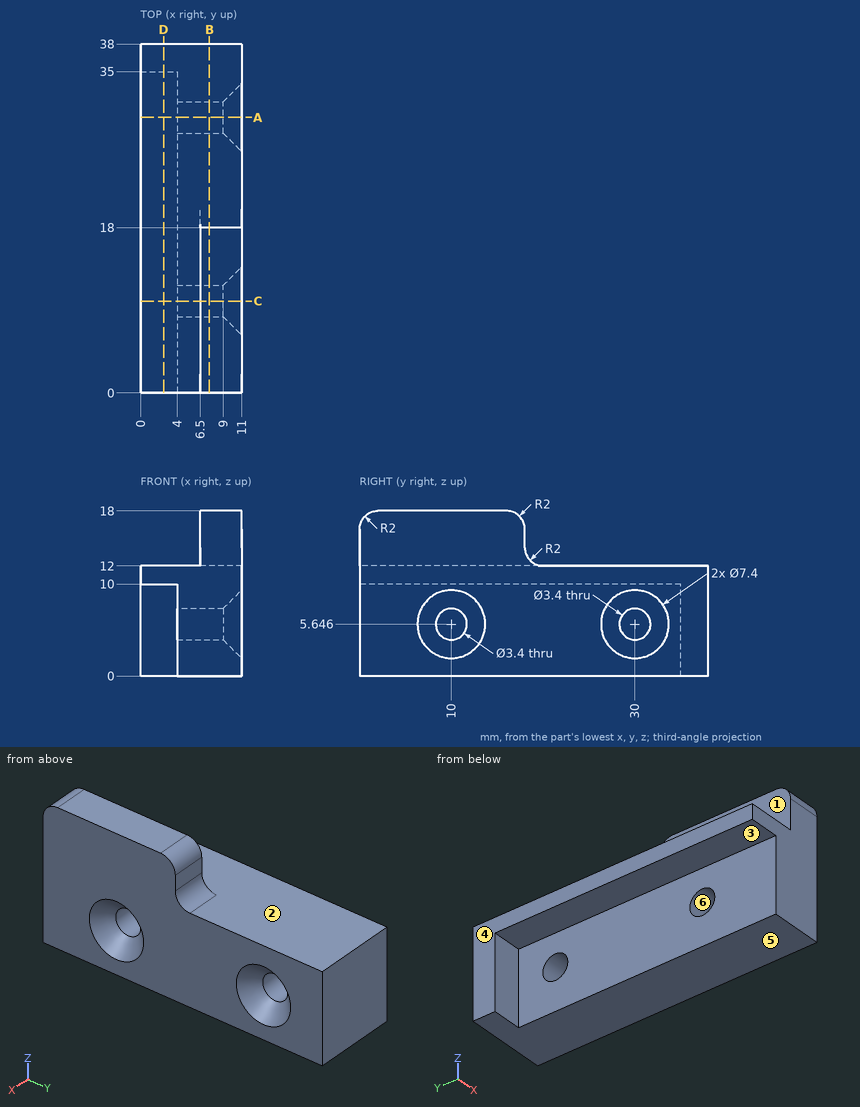
Geometry: see drawing. Coordinates: mm, zero at the bounding-box minimum. A direction names the side the tool comes from. Coordinates: 2 decimals unless noted, no trailing zeros. Loops run counter-clockwise (first coordinate to the right, second up) from the corner with the lowest first, then second, coordinate; pieces in that order, holes last. Notation, with made-up numbers: M 35.25,55 L 82.25,55 A22 ccw 82.25,67 Z; hole C 51,-34 d3. An arc over 180 degrees is marked long. Answer in a Markdown table with one row per item.
Q1. Set-up query: the marked faces 1, 2 and 3. Return all of +Z, -Z, +X, -X, +Y, -Y with unobstructed straight access to the full face (end or side cutting, diameter ignored); none if empty.
Answers below:
| item | result |
|---|---|
| face 1 | +Z, -X, +Y, -Y |
| face 2 | +Z, -X, +Y |
| face 3 | -Z, -X, -Y |
Q2. Section B-B on x = 7.5. Return the cut outline in (y, z) (1 decimal).
Answers below:
| item | result |
|---|---|
| outline | M 0,0 L 38,0 L 38,12 L 20,12 A2 cw 18,14 L 18,16 A2 ccw 16,18 L 2,18 A2 ccw 0,16 Z; hole C 10,5.6 d3.4; hole C 30,5.6 d3.4 |
Q3. Section D-D on x = 2.5. Return the cut outline in (y, z).
Answers below:
| item | result |
|---|---|
| outline | M 0,10 L 35,10 L 35,0 L 38,0 L 38,12 L 0,12 Z |
Q4. Ray query, probe 1 along Z at (x, y) = (7.25, 30) (1 decimal); probe 2 along Z at (x, y) = (6.55, 10) (1 decimal); probe 3 along Z at (x, y) = (4.25, 21.5). Return the intervals inside material, ascending. Write a range as from..to.
Answers below:
| item | result |
|---|---|
| probe 1 | z = 0..3.9, 7.3..12 |
| probe 2 | z = 0..3.9, 7.3..18 |
| probe 3 | z = 0..12 |
Q5. First-contact query: pin 1 (0.6 mm diameter, centred on x = 8, z = 15, fed in from +Y); pin 2 (1.8 mm diameter, centred on y = 10, z = 14, fed in from -X); pin 3 (4 mm diameter, centred on y = 21, z = 6, fed in from -X). Flat tips, straight axial feed; report the tip coordinate or a pass-through.
Answers below:
| item | result |
|---|---|
| pin 1 | stops at y = 18 |
| pin 2 | stops at x = 6.5 |
| pin 3 | stops at x = 4 |
Q6. Draft query along Z for the marked faces 4, 5 and 6. Return one class per face: pulls with the +Z half, pulls with the -Z half, needs draft (parallel to the pull), parting line crosses it, or undercut.
Answers below:
| item | result |
|---|---|
| face 4 | needs draft |
| face 5 | pulls with the -Z half |
| face 6 | undercut |
Q7. Section C-C on y = 10. Return the cut outline in (x, z) (1 decimal).
Answers below:
| item | result |
|---|---|
| outline | M 0,10 L 4,10 L 4,7.3 L 9,7.3 L 11,9.3 L 11,18 L 6.5,18 L 6.5,12 L 0,12 Z; M 4,0 L 11,0 L 11,1.9 L 9,3.9 L 4,3.9 Z |
Q8. Section A-A on y = 30. Return the cut outline in (x, z) (1 decimal).
Answers below:
| item | result |
|---|---|
| outline | M 0,10 L 4,10 L 4,7.3 L 9,7.3 L 11,9.3 L 11,12 L 0,12 Z; M 4,0 L 11,0 L 11,1.9 L 9,3.9 L 4,3.9 Z |
